```python
from build123d import *

# Parameters (mm, degrees)
F1_DEPTH = 60
F2_SIZE  = 5
F3_R     = 25
F4_DEPTH = 25


with BuildPart() as f1:
    # F0 (on Front) → F1 (new body)
    with BuildSketch(Plane.XZ):
        with BuildLine():
            Line((33.428539, 87.827305), (-16.571461, 87.827305))
            ThreePointArc((-16.571461, 87.827305), (-34.24913, 80.504975), (-41.571461, 62.827305))
            Line((-41.571461, 62.827305), (-41.571461, 12.827305))
            ThreePointArc((-41.571461, 12.827305), (-34.24913, -4.850364), (-16.571461, -12.172695))
            Line((-16.571461, -12.172695), (33.428539, -12.172695))
            ThreePointArc((33.428539, -12.172695), (51.106209, -4.850364), (58.428539, 12.827305))
            Line((58.428539, 12.827305), (58.428539, 62.827305))
            ThreePointArc((58.428539, 62.827305), (51.106209, 80.504975), (33.428539, 87.827305))
        make_face()
    extrude(amount=F1_DEPTH)

    # F2
    f2_edges = [f1.edges().sort_by_distance(p)[0] for p in [
        (58.428539, -60, 37.827305),
        (51.106209, -60, 80.504975),
        (8.428539, -60, 87.827305),
        (-34.24913, -60, 80.504975),
        (-41.571461, -60, 37.827305),
        (-34.24913, -60, -4.850364),
        (8.428539, -60, -12.172695),
        (51.106209, -60, -4.850364),
        (58.428539, 0, 37.827305),
        (51.106209, 0, 80.504975),
        (8.428539, 0, 87.827305),
        (-34.24913, 0, 80.504975),
        (-41.571461, 0, 37.827305),
        (-34.24913, 0, -4.850364),
        (8.428539, 0, -12.172695),
        (51.106209, 0, -4.850364),
    ]]
    chamfer(f2_edges, length=F2_SIZE)

    # F3 (on face) → F4 (cut)
    with BuildSketch(Plane.XZ.offset(60)):
        with Locations((5.020919, 40.530141)):
            Circle(F3_R)
    extrude(amount=-F4_DEPTH, mode=Mode.SUBTRACT)


solid = f1.part
```
For this review, take the finished solid that the model builds, in its own axes (mm). Give positions to 0.01 mm unless a question says otherwise; leave off trailing zeros. Write each loop counter-clockwise with the first axis right and the second up, starting at its lowest first coordinate (ties: lowest second). Pieces come first, ordered by that corner, then holes. Notation, with made-up numbers: M 39.5,50.5 L 74.5,50.5 A28 ccw 74.5,80.5 Z; hole C 33,81.5 d2. An arc over 180 degrees is marked long. Answer as a JSON object with one key per item and string values. Group by question number.
Item 1: Consider section D-D on z = 29. Write out the cut boundary in (x, y).
Item 2: For pin 1 Ø1.5 at (x, y) = (-28.5, -25.5) entering from +Z; pin 2 Ø3 at (y, z) = (-45, 2) entering from +X; pin 3 Ø1.5 at (x, y) = (-19, -42) entering from -Z, all flat-tipped, find the tip position at first contact; note any pin that passes through.
Item 3: Consider section C-C on y = -51. Write out the cut boundary in (x, z).
Item 4: Consider section A-A on y = -21. Write out the cut boundary in (x, z).
Item 5: Consider section B-B on x = -8. Write out the cut boundary in (y, z), plus the area to 3 significant figures.
Item 6: For probe 1 along X at (y, z) = (-43.5, 41); probe 2 along Y at (x, z) = (29.5, 42.5); probe 3 along X at (y, z) = (-18, 12), list the stretches that pass through material, from the lowest coordinate up. Write a range as [from, to].
Check result:
{
 "1": {"outline": "M -41.57,-55 L -36.57,-60 L -17.16,-60 L -17.16,-35 L 27.2,-35 L 27.2,-60 L 53.43,-60 L 58.43,-55 L 58.43,-5 L 53.43,0 L -36.57,0 L -41.57,-5 Z"},
 "2": {"pin 1": "stops at z = 85.19", "pin 2": "stops at x = 56.62", "pin 3": "stops at z = -12.12"},
 "3": {"outline": "M -41.57,12.83 A25 ccw -16.57,-12.17 L 33.43,-12.17 A25 ccw 58.43,12.83 L 58.43,62.83 A25 ccw 33.43,87.83 L -16.57,87.83 A25 ccw -41.57,62.83 Z; hole C 5.02,40.53 d50"},
 "4": {"outline": "M -41.57,12.83 A25 ccw -16.57,-12.17 L 33.43,-12.17 A25 ccw 58.43,12.83 L 58.43,62.83 A25 ccw 33.43,87.83 L -16.57,87.83 A25 ccw -41.57,62.83 Z"},
 "5": {"outline": "M -60,-7.17 L -55,-12.17 L -5,-12.17 L 0,-7.17 L 0,82.83 L -5,87.83 L -55,87.83 L -60,82.83 L -60,61.87 L -35,61.87 L -35,19.19 L -60,19.19 Z", "area": "4,880 mm^2"},
 "6": {"probe 1": "x = [-41.57, -19.97], [30.02, 58.43]", "probe 2": "y = [-35, 0]", "probe 3": "x = [-41.56, 58.41]"}
}
